Job drawing, mm, ordinate dimensions from the low corner. One solid piece. A direction names the side the tool comes from. Coordinates: 2 decimals unless noted, no trailing zeros. Order: outer loops, then holes, each group sorted by start corner. A loop starts at its lowest first (then second) coordinate and runs counter-clockwise, first axis right, second up. Notation, with made-up numbers: (80.25, -19.75) - (109.25, -19.75) arc R23 cw to (109.25, -4.75) - close; hole circle Ø2 at (-22, -6.75). An arc over 180 degrees is marked (long way). Write each question's results on one line, items separated by ' | '. Start each with the question number.
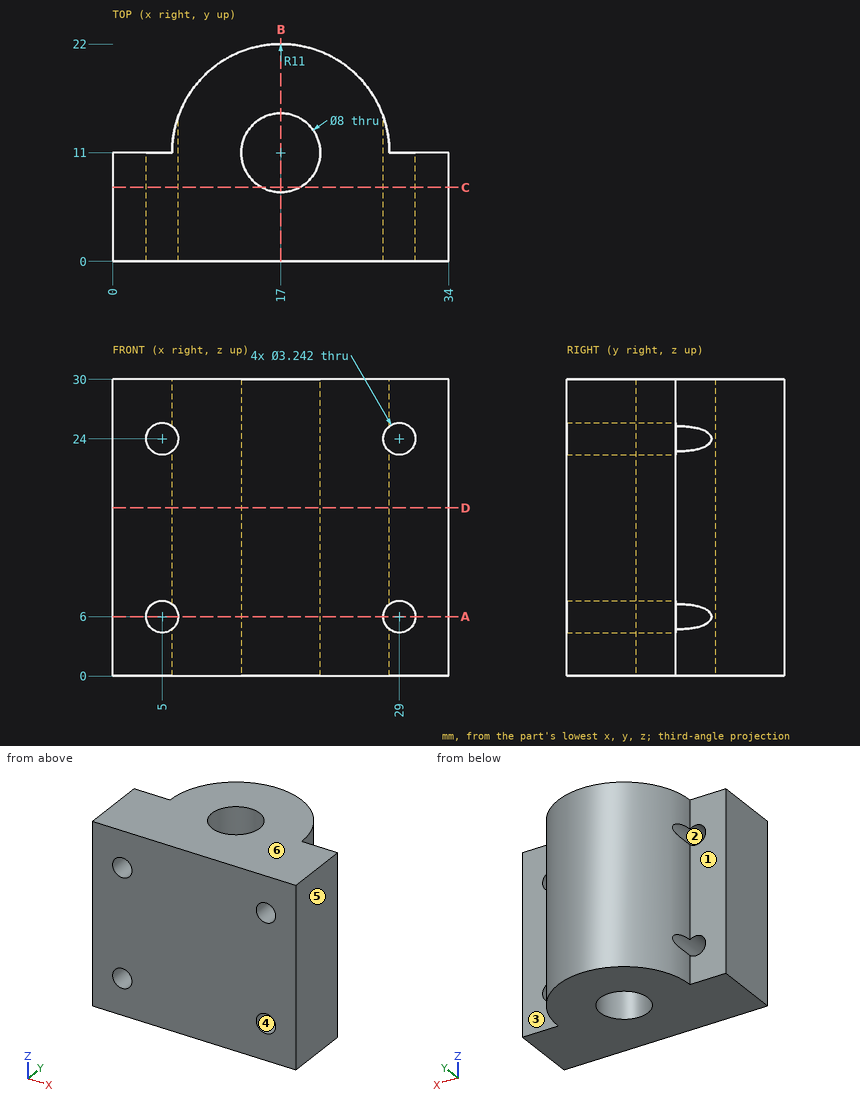
Item 1: Probe probe 1 along X at (y, z) = (6.25, 6); probe 2 along Z at (x, y) = (5, 9.5); probe 3 along Y at (x, z) = (17, 24.5). List the from-to ranges inside material, lowest first.
Item 2: Slice it at D-D (z = 17). Write the cut outline in (x, y).
Item 3: Flat gauge pins, fed straight in: P1, Ø1.8, axis at x = 31, z = 18.5, coming from the +Y side; P2, Ø4, axis at x = 6, z = 8.5, coming from the +Y side; P3, Ø3, axis at x = 5, z = 24, coming from the -Y side; P4, Ø5, axis at y = 15.5, z = 26, coming from the +X side. Where does each tip first touch, or does it go through?
Item 4: Slice it at B-B (x = 17). Write the cut outline in (y, z).
Item 5: Slice it at C-C (y = 7.5). Write the cut outline in (x, z).
Item 6: Slice it at A-A (z = 6). Write the cut outline in (x, y), then the cut area to 3 significant figures.
Item 7: Pull direction Z, two halves, no side cores. Call the marked faces 4, 5 and 6: released by +Z, released by -Z, zero draft, split by the parting line, or undercut.
Item 8: Which spindle directions (+Z, -Z, +X, -X, +Y, -Y) get a long thin tool onto all of the face, cutting with end or side? Do the marked faces 1, 2 and 3. Say none if no direction does.
Resolved:
1) probe 1: 0 to 3.38, 6.62 to 27.38, 30.62 to 34 | probe 2: 0 to 4.38, 7.62 to 22.38, 25.62 to 30 | probe 3: 0 to 7, 15 to 22
2) outline: (0, 0) - (34, 0) - (34, 11) - (28, 11) arc R11 ccw to (6, 11) - (0, 11) - close; hole circle Ø8 at (17, 11)
3) P1: y = 11 | P2: y = 17.32 | P3: through | P4: x = 27.82
4) outline: (0, 0) - (7, 0) - (7, 30) - (0, 30) - close; (15, 0) - (22, 0) - (22, 30) - (15, 30) - close
5) outline: (0, 0) - (15.06, 0) - (15.06, 30) - (0, 30) - close; (18.94, 0) - (34, 0) - (34, 30) - (18.94, 30) - close; hole circle Ø3.24 at (5, 6); hole circle Ø3.24 at (5, 24); hole circle Ø3.24 at (29, 6); hole circle Ø3.24 at (29, 24)
6) outline: (0, 0) - (3.38, 0) - (3.38, 11) - (0, 11) - close; (6.62, 0) - (27.38, 0) - (27.38, 14.64) arc R11 ccw to (6.62, 14.64) - close; (30.62, 0) - (34, 0) - (34, 11) - (30.62, 11) - close; hole circle Ø8 at (17, 11) | area: 439 mm^2
7) face 4: undercut | face 5: zero draft | face 6: released by +Z
8) face 1: +Z, -Z, -X, +Y | face 2: +Y, -Y | face 3: +Z, -Z, +X, +Y
